Can you work these out from the model? Positions are in its coordinate system, mm. A direction names the side the tool comes from. Round coordinates to 2 decimals unless told otherwise and drop trailing zeros. Write each loop counter-clockwise with the first axis right and the second up, starting at its lowest first coordinate (ties: lowest second). Pieces come first, ordered by that corner, then holes. Notation, with made-up numbers: M 56,49 L 64,49 A18 cw 64,60 Z; hole C -33.5,5 d11. An arc over 180 degrees is marked long. Use one line per item in the form item = value. Start each with the question number.
```python
from build123d import *

# Parameters (mm, degrees)
SKETCH1_R                     = 10
BOSS_EXTRUDE1_DEPTH           = 5
CBORE_FOR_M3_SHCS1_AT_2_COUNT = 2
CBORE_FOR_M3_SHCS1_AT_2_PITCH = 7.52
CHAMFER1_SIZE                 = 0.4


with BuildPart() as part:
    # Sketch1 → Boss-Extrude1 (new body)
    with BuildSketch(Plane(origin=(0, 0, 0), x_dir=(1, 0, 0), z_dir=(0, 1, 0))):
        with Locations(Location((0, 0, 0), (0, 0, 270))):
            Circle(SKETCH1_R)
    extrude(amount=BOSS_EXTRUDE1_DEPTH)

    # Sketch3 → CBORE for M3 SHCS1 (revolve, cut)
    with BuildSketch(Plane(origin=(0, 5, -3.76), x_dir=(0, 0, 1), z_dir=(1, 0, 0))):
        Polygon((0, 0), (0, 5), (2.1, 5), (1.7, 4.6), (1.7, 3.4), (2.1, 3), (3.25, 3), (3.25, 0.4), (3.65, 0), align=None)
    cbore_for_m3_shcs1 = revolve(axis=Axis((0, 11.35, -3.76), (0, -1, 0)), mode=Mode.SUBTRACT)

    # CBORE for M3 SHCS1 at 2: CBORE for M3 SHCS1 ×2
    with Locations(*[(0, 0, i * CBORE_FOR_M3_SHCS1_AT_2_PITCH) for i in range(1, CBORE_FOR_M3_SHCS1_AT_2_COUNT)]):
        add(cbore_for_m3_shcs1, mode=Mode.SUBTRACT)

    # Chamfer1
    chamfer1_edges = [part.edges().sort_by_distance(p)[0] for p in [
        (0, 0, -10),
        (0, 5, -10),
    ]]
    chamfer(chamfer1_edges, length=CHAMFER1_SIZE)


solid = part.part
```
1. If we section it at C-C (y = 2.55): List the corners of the cut face in (x, z) for me, and give its area (3 significant figures).
2. Will these pins go through, and if not, where does the flat tip stop? pin 1 (1.5 mm diameter, centred on x = 5.5, y = 1, fed in from +Z); pin 2 (5.5 mm diameter, centred on x = 0, z = 3.76, fed in from +Y); pin 3 (4 mm diameter, centred on x = 0, z = -3.76, fed in from -Y).
3. If we section it at A-A (y = 0.75): List the corners of the cut face in (x, z) for me, and give its area (3 significant figures).
4. Please list where these lines run through material, in increasing order: line 1 along Z through (x, y) = (-0.25, 0.3); line 2 along X through (y, z) = (2.6, 4.75); line 3 along Z through (x, y) = (2.25, 2.95).
5. If we mould it in two halves opening along X, with no side actions, what happens to faces 1 (the face through (0, 0, 0)), 2 (the face through (-9.76, 2.47, -2.17)), 3 (the face through (2, 3.3, 1.2)), 4 (the face through (1.66, 1.01, -4.13))? For each: pulls with the +X half, pulls with the -X half, needs draft (parallel to the pull), parting line crosses it, or undercut.
6. Which directions (+Z, -Z, +X, -X, +Y, -Y) give clear straight access to the entire face, cutting with the end or side of a thin tool? Please do faces 5 (the face through (-2, 5, 0)), 6 (the face through (1, 2, -6)).
7. If we section it at B-B (x = 0): State how many separate pieces and enclosed holes the cut face has, and give its area (3 significant figures).
Model answer:
q1.outline = C 0,0 d20; hole C 0,-3.76 d6.5; hole C 0,3.76 d6.5
q1.area = 248 mm2
q2.pin_1 = 8.8
q2.pin_2 = 2
q2.pin_3 = 0.1
q3.outline = C 0,0 d20; hole C 0,-3.76 d3.4; hole C 0,3.76 d3.4
q3.area = 296 mm2
q4.line_1 = -9.9 to -5.54, -1.98 to 1.98, 5.54 to 9.9
q4.line_2 = -8.8 to -3.1, 3.1 to 8.8
q4.line_3 = -9.74 to -6.11, -1.41 to 1.41, 6.11 to 9.74
q5.face_1 = needs draft
q5.face_2 = parting line crosses it
q5.face_3 = undercut
q5.face_4 = undercut
q6.face_5 = +Z, -Z, +X, -X, +Y
q6.face_6 = +Y
q7.separate_pieces = 3
q7.enclosed_holes = 0
q7.area = 46.1 mm2
